from build123d import *

# Parameters (mm, degrees)
F0_R            = 50
F0_R_2          = 25
F1_DEPTH        = 20
F2_R            = 6
F3_DEPTH        = 25
F3_COPIES_COUNT = 5


# Not quite as in the source:
# - a pattern or mirror of a feature is missing from the dataset's text; its kind, count and spacing are read off the source's solid


with BuildPart() as f1:
    # F0 (on Front) → F1 (new body)
    with BuildSketch(Plane.XZ):
        Circle(F0_R)
        Circle(F0_R_2, mode=Mode.SUBTRACT)
    extrude(amount=F1_DEPTH)

    # F2 (on face) → F3 (cut)
    with BuildSketch(Plane.XZ.offset(20)):
        with Locations((0, 37.5)):
            Circle(F2_R)
    f3 = extrude(amount=-F3_DEPTH, mode=Mode.SUBTRACT)

    # F3_copies: F3 ×5 about axis
    f3_copies_axis = Axis((0, 0, 0), (0, 1, 0))
    for i in range(1, F3_COPIES_COUNT):
        add(f3.rotate(f3_copies_axis, i * 360 / F3_COPIES_COUNT), mode=Mode.SUBTRACT)


solid = f1.part
Source: CAD feature listing. Evaluate the final solid. Frame: model axes, mm. Round coordinates to 2 decimals unless told otherwise and drop trailing zeros. Write each loop counter-clockwise with the first axis right and the second up, starting at its lowest first coordinate (ties: lowest second). Pieces come first, ordered by that corner, then holes. Notation, with made-up numbers: M 0.5,88.25 L 30.5,88.25 A21 cw 30.5,94.25 Z; hole C -22.5,65.5 d6. An arc over 180 degrees is marked long. One line per item, written item: value. Start each with the question number.
Item 1: Section query A-A (x = 0). Return the cut outline in (y, z), plus the area to 3 significant figures.
Item 2: Ray query, L1, parallel to Z at x = 0.5, y = -11.5 (1 decimal); L2, parallel to X at y = -8.5, z = -0.5 (1 decimal); L3, parallel to Z at x = -18.5, y = -4.75. Return the intervals inside material, ascending. Write a range as from..to.
Item 3: Mould query, pull axis Z, two halves, no side actions, for faces 1 (the cylindrical face through (47.69, -9.86, 15.02)), 2 (the cylindrical face through (-1.301, -10.14, 31.643)), 3 (the cylindrical face through (-24.91, -10.14, -35.61)), 4 (the flat face through (10.4, -20, 22.9)). Classes: pulls with the +Z half, pulls with the -Z half, needs draft (parallel to the pull), parting line crosses it, or undercut.
Item 4: Section query D-D (x = -39.5). Return the cut outline in (y, z), plus the area to 3 significant figures.
Item 5: Section query C-C (y = -11). Return the cut outline in (x, z), plus the area to 4 significant figures.
Item 6: Pin query (flat end, axial travel): pin 1 (3 mm diameter, centred on x = -27, z = -21.5, fed in from +Y); pin 2 (3 mm diameter, centred on x = -24, y = -16, fed in from -Z); pin 3 (5 mm diameter, centred on y = -6.5, z = 26, fed in from +X); pin 4 (11 mm diameter, centred on x = 0, z = 37.5, fed in from -Y). Return the tip coordinate at first contact, or that it passes through.
Item 7: Section query B-B (z = 0). Return the cut outline in (x, y).
Result set:
1. outline: M -20,-50 L 0,-50 L 0,-25 L -20,-25 Z; M -20,25 L 0,25 L 0,31.5 L -20,31.5 Z; M -20,43.5 L 0,43.5 L 0,50 L -20,50 Z
1. area: 760 mm²
2. L1: z = -50..-25, 25..31.5, 43.5..50
2. L2: x = -50..-25, 25..50
2. L3: z = -46.45..-35.18, -25.5..-16.82, 16.82..46.45
3. face 1: parting line crosses it
3. face 2: undercut
3. face 3: undercut
3. face 4: needs draft
4. outline: M -20,-30.66 L 0,-30.66 L 0,6.97 L -20,6.97 Z; M -20,16.2 L 0,16.2 L 0,30.66 L -20,30.66 Z
4. area: 1,040 mm²
5. outline: C 0,0 d100; hole C -35.66,11.59 d12; hole C -22.04,-30.34 d12; hole C 0,0 d50; hole C 0,37.5 d12; hole C 22.04,-30.34 d12; hole C 35.66,11.59 d12
5. area: 5,325 mm²
6. pin 1: stops at y = 0
6. pin 2: stops at z = -44.65
6. pin 3: stops at x = 44.13
6. pin 4: passes through
7. outline: M -50,-20 L -25,-20 L -25,0 L -50,0 Z; M 25,-20 L 50,-20 L 50,0 L 25,0 Z
